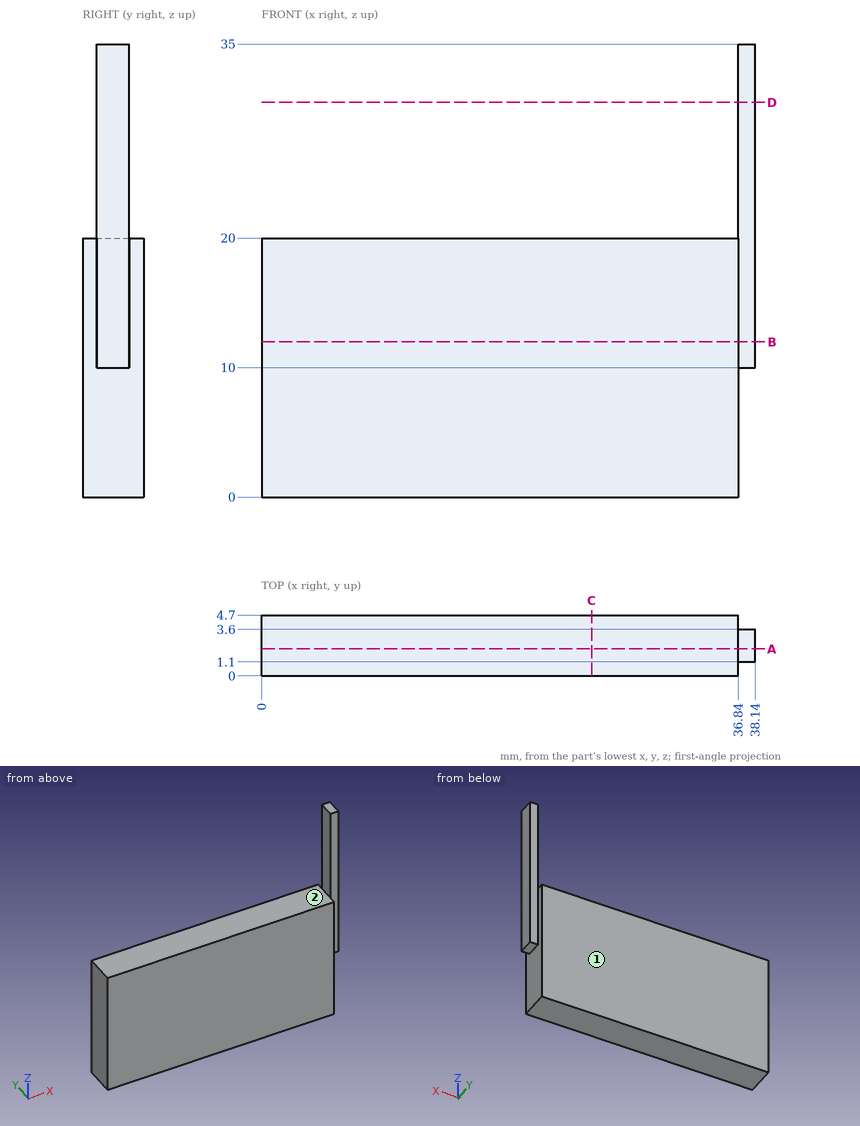
For this review, use the dimensioned drawing (mm, ordinates from the lowest corner) and the shaded views. A direction names the side the tool comes from. Coordinates: 2 decimals unless noted, no trailing zeros. Loops run counter-clockwise (first coordinate to the right, second up) from the corner with the lowest first, then second, coordinate; pieces in that order, holes last. Notation, with made-up numbers: (42, 50.5) -> (98, 50.5) arc R13 ccw to (98, 72.5) -> close; hole circle Ø2 at (82.25, 58.5). An arc over 180 degrees is marked (long way). Use a Markdown table: item, result. Add a question column.
1. Add section B-B on z = 12. Write out the cut boundary in (x, y).
2. Add section A-A on y = 2.1. Write out the cut boundary in (x, z).
3. Machinability: for the marked faces 1 and 2, which of the approach directions +Z, -Z, +X, -X, +Y, -Y give a long, thin tool a straight path to every point of the face, cutting with its end or side? Answer none if there is none.
4. Add section D-D on z = 30.5. Write out the cut boundary in (x, y), plus the area to 3 significant figures.
5. To check wall thickness, follow line 1 (X direction, y = 2.25, z = 4); line 2 (Z direction, x = 9, y = 0.6); line 3 (X direction, y = 3.45, z = 28.5). State the ranges of each line that lie inside material, in increasing order.
6. Clearance check with flat-ended pins moving along their axes: pin 1 Ø1 at (x, z) = (37.5, 19.5) entering from -Y; pin 2 Ø1.4 at (x, y) = (21, 2.5) entering from +Z. State where each tip first meets the part, or that it passes through.
7. Add section C-C on x = 25.5. Write out the cut boundary in (y, z), plus the area to 3 significant figures.
Returned:
| question | item | result |
|---|---|---|
| 1 | outline | (0, 0) -> (36.84, 0) -> (36.84, 1.1) -> (38.14, 1.1) -> (38.14, 3.6) -> (36.84, 3.6) -> (36.84, 4.7) -> (0, 4.7) -> close |
| 2 | outline | (0, 0) -> (36.84, 0) -> (36.84, 10) -> (38.14, 10) -> (38.14, 35) -> (36.84, 35) -> (36.84, 20) -> (0, 20) -> close |
| 3 | face 1 | +Z, -Z, +X, -X, +Y |
| 3 | face 2 | +Z, -X, +Y, -Y |
| 4 | outline | (36.84, 1.1) -> (38.14, 1.1) -> (38.14, 3.6) -> (36.84, 3.6) -> close |
| 4 | area | 3.25 mm² |
| 5 | line 1 | x = 0 to 36.84 |
| 5 | line 2 | z = 0 to 20 |
| 5 | line 3 | x = 36.84 to 38.14 |
| 6 | pin 1 | stops at y = 1.1 |
| 6 | pin 2 | stops at z = 20 |
| 7 | outline | (0, 0) -> (4.7, 0) -> (4.7, 20) -> (0, 20) -> close |
| 7 | area | 94.0 mm² |
